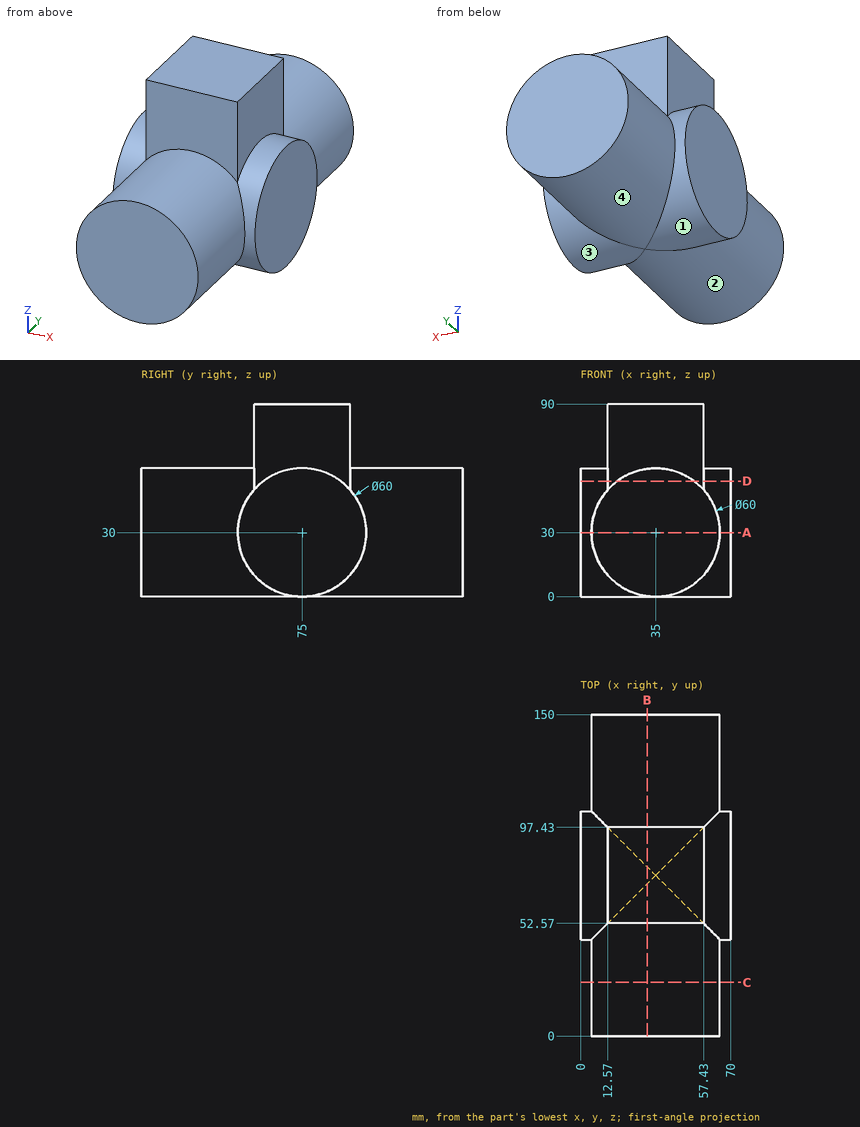
The figure shows three views and two pictorial views of one solid part (mm, origin at its lowest corner). Answer the questions. A direction names the side the tool comes from. Coordinates: 2 decimals unless noted, no trailing zeros. Loops run counter-clockwise (first coordinate to the right, second up) from the corner with the lowest first, then second, coordinate; pieces in that order, holes last. Notation, with made-up numbers: (-26, -2) -> (-21, -2) arc R17 ccw to (-21, 6) -> close; hole circle Ø7 at (36, 64.25). An arc over 180 degrees is marked (long way). Return JSON: item names as keys, results as strings. Group by question number.
(1) A cutting plane is placed at B-B on x = 31. Write down the section's boundary in (y, z), and give its area (3 significant figures).
(2) A cutting plane is placed at D-D on z = 54. Write down the section's boundary in (x, y), and give its area (3 significant figures).
(3) Which of the six approach directions +Z, -Z, +X, -X, +Y, -Y give full straight-line access (tool end or side, diameter ignored) to the marked faces 1, 2, 3 and 4?
(4) Find the intervals of material crossed by probe 1 along Z at (x, y) = (42.5, 74); probe 2 along Y at (x, z) = (25, 78); probe 3 along X at (y, z) = (69, 74), in increasing order. Write a range as from..to.
(5) Given pin 1 Ø8 at (x, y) = (19, 55) entering from -Z (1 decimal); pin 2 Ø1 at (x, y) = (7, 97.5) entering from -Z; pin 3 Ø6 at (y, z) = (114, 15) entering from -X (1 decimal), each flat-ended and moving along its own axis, determine where each tip first touches the part or whether it passes through.
(6) A cutting plane is placed at A-A on z = 30. Write down the section's boundary in (x, y), and give its area (3 significant figures).
(7) A cutting plane is placed at C-C on y = 25. Write down the section's boundary in (x, z).
The answers:
{
 "1": {"outline": "(0, 0.27) -> (71, 0.27) arc R30 ccw to (79, 0.27) -> (150, 0.27) -> (150, 59.73) -> (97.43, 59.73) -> (97.43, 90) -> (52.57, 90) -> (52.57, 59.73) -> (0, 59.73) -> close", "area": "10,300 mm^2"},
 "2": {"outline": "(0, 57) -> (12.57, 57) -> (12.57, 52.57) -> (17, 52.57) -> (17, 0) -> (53, 0) -> (53, 52.57) -> (57.43, 52.57) -> (57.43, 57) -> (70, 57) -> (70, 93) -> (57.43, 93) -> (57.43, 97.43) -> (53, 97.43) -> (53, 150) -> (17, 150) -> (17, 97.43) -> (12.57, 97.43) -> (12.57, 93) -> (0, 93) -> close", "area": "6,700 mm^2"},
 "3": {"face 1": "-X", "face 2": "-Y", "face 3": "+X", "face 4": "+Y"},
 "4": {"probe 1": "z = 0.02..90", "probe 2": "y = 52.57..97.43", "probe 3": "x = 12.57..57.43"},
 "5": {"pin 1": "stops at z = 2.5", "pin 2": "stops at z = 9.6", "pin 3": "stops at x = 7.5"},
 "6": {"outline": "(0, 45) -> (5, 45) -> (5, 0) -> (65, 0) -> (65, 45) -> (70, 45) -> (70, 105) -> (65, 105) -> (65, 150) -> (5, 150) -> (5, 105) -> (0, 105) -> close", "area": "9,600 mm^2"},
 "7": {"outline": "circle Ø60 at (35, 30)"}
}
